Geometry check sheet. Reference: drawing and pictorial views, mm from the part's lowest x, y, z. Coordinates: 2 decimals unless noted, no trailing zeros. Loops run counter-clockwise (first coordinate to the right, second up) from the corner with the lowest first, then second, coordinate; pieces in that order, holes last.
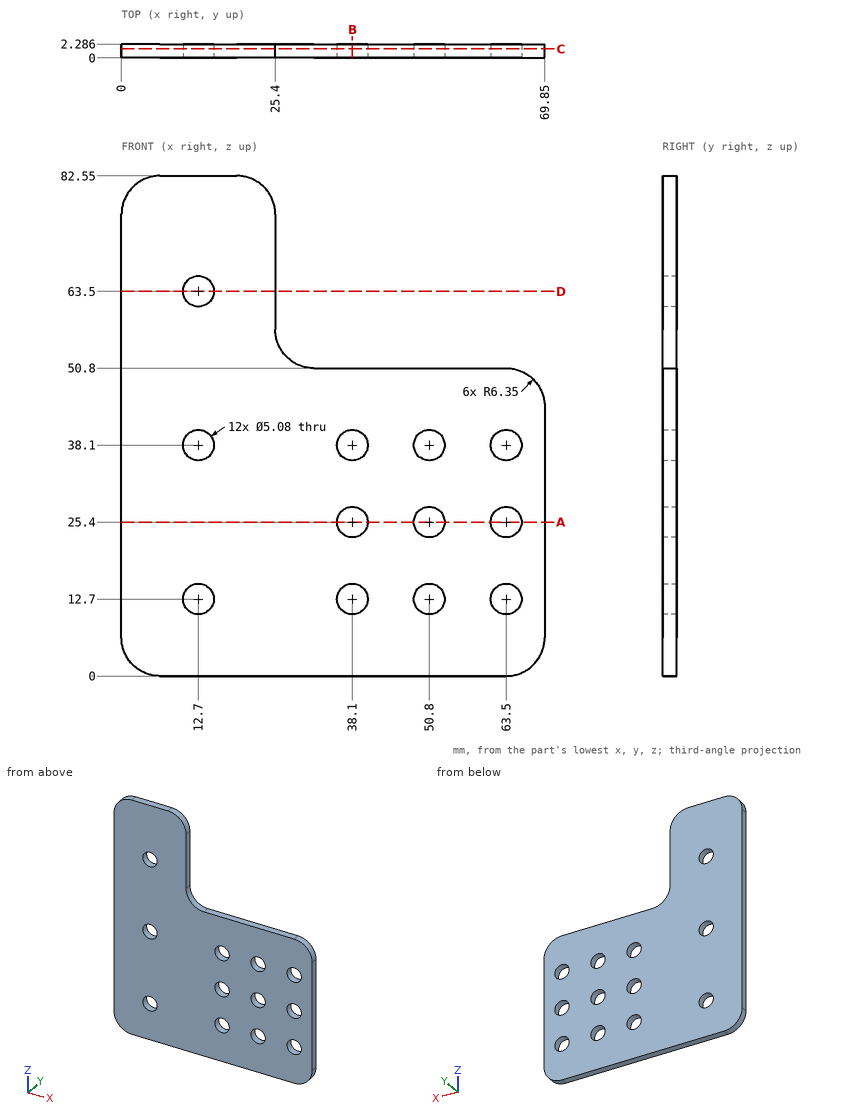
1) Depth check by flat-ended pin: pin 1 (6 mm diameter, centred on x = 63.5, z = 38.1, fed in from +Y); pin 2 (0.7 mm diameter, centred on x = 52, y = 1, fed in from +Z); pin 3 (1.1 mm diameter, centred on y = 1.5, z = 62.5, fed in from +X). Enter the tip coordinate at first touch or a pass-through.
Data:
pin 1: stops at y = 2.29
pin 2: stops at z = 50.8
pin 3: stops at x = 25.4
2) Section check A-A on z = 25.4. Record the cut outline in (x, y).
Data:
outline: (0, 0) - (35.56, 0) - (35.56, 2.29) - (0, 2.29) - close; (40.64, 0) - (48.26, 0) - (48.26, 2.29) - (40.64, 2.29) - close; (53.34, 0) - (60.96, 0) - (60.96, 2.29) - (53.34, 2.29) - close; (66.04, 0) - (69.85, 0) - (69.85, 2.29) - (66.04, 2.29) - close
3) Section check D-D on z = 63.5. Record the cut outline in (x, y), and give its area (3 significant figures).
Data:
outline: (0, 0) - (10.16, 0) - (10.16, 2.29) - (0, 2.29) - close; (15.24, 0) - (25.4, 0) - (25.4, 2.29) - (15.24, 2.29) - close
area: 46.5 mm2
4) Material ranges on probe 1 along X at (y, z) = (1.45, 12.7); probe 2 along X at (y, z) = (2.1, 10.5); probe 3 along X at (y, z) = (0.85, 25.4), recorded low to high.
Data:
probe 1: x = 0 to 10.16, 15.24 to 35.56, 40.64 to 48.26, 53.34 to 60.96, 66.04 to 69.85
probe 2: x = 0 to 11.43, 13.97 to 36.83, 39.37 to 49.53, 52.07 to 62.23, 64.77 to 69.85
probe 3: x = 0 to 35.56, 40.64 to 48.26, 53.34 to 60.96, 66.04 to 69.85
5) Section check B-B on x = 38.1. Record the cut outline in (y, z).
Data:
outline: (0, 0) - (2.29, 0) - (2.29, 10.16) - (0, 10.16) - close; (0, 15.24) - (2.29, 15.24) - (2.29, 22.86) - (0, 22.86) - close; (0, 27.94) - (2.29, 27.94) - (2.29, 35.56) - (0, 35.56) - close; (0, 40.64) - (2.29, 40.64) - (2.29, 50.8) - (0, 50.8) - close
6) Section check C-C on y = 1.5. Count the separate pieces of the cut face and the enclosed holes in it, and give its area (3 significant figures).
Data:
separate pieces: 1
enclosed holes: 12
area: 4,080 mm2
